Can you work these out from the model? Positions are in its coordinate system, mm. A direction names the side the tool comes from. Coordinates: 2 decimals unless noted, no trailing zeros. Loops run counter-clockwise (first coordinate to the right, second up) from the corner with the lowest first, then second, coordinate; pieces in that order, holes last. Notation, with made-up numbers: (26, 39) -> (74, 39) arc R24 ccw to (74, 50) -> close; hole circle Ø9 at (59.25, 25). An arc over 180 degrees is marked (long way). Use one line per item in the form item = value. Start each with the question number.
(1) I'm going to push flat-ended pins straight in: pin 1 (8 mm diameter, centred on y = -72, z = 7, fed in from +X); pin 2 (6 mm diameter, centred on y = -24.5, z = -0.5, fed in from -X) (3 decimals); pin 3 (4 mm diameter, centred on x = 6, y = -33.5, fed in from +Z). Where does each tip first touch, or does it pass through?
(2) On a 3-axis mill with a long thin cutter (end or side, diameter ignored), from which of +Z, -Z, +X, -X, +Y, -Y can I reach the whole of each face in a straight line? I mean faces 1 (the flat face through (0, 0, 0)), 2 (the cylindrical face through (4.44, -53.29, 6.96)). Say none if no direction works.
(3) Imagine slicing it at B-B (x = 0). List the corners of the cut face in (y, z) for me (3 decimals).
(4) Imagine slicing it at A-A (z = 0). List the corners of the cut face in (x, y) for me (3 decimals).
(5) I need wall thicknesses on line 1 (Z direction, x = 0, y = -6.5) (3 decimals); line 2 (X direction, y = -111, z = -2.75); line 3 (X direction, y = -116, z = 6.25). Which ranges of each line are inside material? Lowest first, please. Write a range as [from, to].
(6) Imagine slicing it at C-C (y = -47). List the corners of the cut face in (x, z) for me (3 decimals), plus the area to 3 significant figures.
```python
from build123d import *

# Parameters (mm, degrees)
F0_R        = 8.255
F1_DEPTH    = 99.06
F2_R        = 9.525
F3_DEPTH    = 25.4
F4_S5_R     = 8.255
F4_T6_DEPTH = 15
F5_SIZE     = 5.08


# Not quite as in the source:
# - a fillet or chamfer that OpenCascade refuses, or shapes differently, is made with other operations: its cross-section is extruded or revolved along the edge and cut away or added


with BuildPart() as f1:
    # F0 (on Front) → F1 (new body)
    with BuildSketch(Plane.XZ):
        Circle(F0_R)
    extrude(amount=F1_DEPTH)

    # F2 (on face) → F3 (join)
    with BuildSketch(Plane.XZ.offset(99.06)):
        Circle(F2_R)
    extrude(amount=F3_DEPTH)

    # F4: chamfer of 5.08 on 3 edges, made by hand


with BuildPart() as f4_tool2:
    # F4_s3 → F4_t4 (revolve)
    with BuildSketch(Plane.XY):
        Polygon((9.525, -104.14), (4.445, -99.06), (9.525, -99.06), align=None)
    revolve(axis=Axis((0, -99.06, 0), (0, -1, 0)))

    # F4_s5 → F4_t6 (cut, symmetric)
    with BuildSketch(Plane.XZ.offset(101.6)):
        Circle(F4_S5_R)
    extrude(amount=F4_T6_DEPTH, both=True, mode=Mode.SUBTRACT)


with BuildPart() as f1_1:
    add(f1.part)

    # F4_t1: cut F4_tool2
    add(f4_tool2.part, mode=Mode.SUBTRACT)

    # F4_s7 → F4_t8 (revolve, cut)
    with BuildSketch(Plane.XY):
        Polygon((9.525, -119.38), (4.445, -124.46), (9.525, -124.46), align=None)
    revolve(axis=Axis((0, -124.46, 0), (0, -1, 0)), mode=Mode.SUBTRACT)

    # F5
    f5_edges = [f1_1.edges().sort_by_distance(p)[0] for p in [
        (-8.255, 0, 0),
    ]]
    chamfer(f5_edges, length=F5_SIZE)


solid = f1_1.part
```
Worked out:
q1.pin_1 = 7.69
q1.pin_2 = -8.255
q1.pin_3 = 7.22
q2.face_1 = +Z, -Z, +X, -X, +Y
q2.face_2 = +Y
q3.outline = (-124.46, -4.445) -> (-119.38, -9.525) -> (-104.14, -9.525) -> (-102.87, -8.255) -> (-5.08, -8.255) -> (0, -3.175) -> (0, 3.175) -> (-5.08, 8.255) -> (-102.87, 8.255) -> (-104.14, 9.525) -> (-119.38, 9.525) -> (-124.46, 4.445) -> close
q4.outline = (-9.525, -119.38) -> (-4.445, -124.46) -> (4.445, -124.46) -> (9.525, -119.38) -> (9.525, -104.14) -> (8.255, -102.87) -> (8.255, -5.08) -> (3.175, 0) -> (-3.175, 0) -> (-8.255, -5.08) -> (-8.255, -102.87) -> (-9.525, -104.14) -> close
q5.line_1 = [-8.255, 8.255]
q5.line_2 = [-9.12, 9.12]
q5.line_3 = [-7.19, 7.19]
q6.outline = circle Ø16.51 at (0, 0)
q6.area = 214 mm2
